Input: part model. Units: mm. Frame: model coordinates. Round coordinates to 2 decimals unless told otherwise and drop trailing zeros. Write each loop counter-clockwise with the first axis right and the second up, starting at its lowest first coordinate (ties: lowest second). Pieces come first, ordered by that corner, then holes. Notation, with made-up numbers: (-29.5, 12) -> (27.5, 12) arc R20 ccw to (27.5, 30) -> close; hole circle Ø11 at (-29.5, 34). An arc over 180 degrees is marked (long way). Use CSV: the item, a comma, the result in double quotes.
```python
from build123d import *

# Parameters (mm, degrees)
F0_W        = 21
F0_H        = 147
F1_DEPTH    = 4
F3_DEPTH    = 4.001
F4_T1_DEPTH = 171.4948974279


# Not quite as in the source:
# - a fillet or chamfer that OpenCascade refuses, or shapes differently, is made with other operations: its cross-section is extruded or revolved along the edge and cut away or added


with BuildPart() as f1:
    # F0 (on Top) → F1 (new body)
    with BuildSketch(Plane.XY):
        Rectangle(F0_W, F0_H)
    extrude(amount=F1_DEPTH)

    # F2 (on face) → F3 (cut, through all)
    with BuildSketch(Plane.XY.offset(4)):
        Polygon((10.5, 73.5), (-10.5, 73.5), (10.5, 52.5), align=None)
        Polygon((10.5, -52.5), (-10.5, -73.5), (10.5, -73.5), align=None)
    extrude(amount=-F3_DEPTH, mode=Mode.SUBTRACT)

    # F4: fillet of radius 5 on 1 edges, made by hand

    # F4_s2 → F4_t1 (cut)
    with BuildSketch(Plane.XZ.offset(-85.7474487139)):
        with BuildLine():
            ThreePointArc((-5.6010205144, 4), (-8.7632981746, 2.8729833462), (-10.5, 0))
            Line((-10.5, 0), (-10.5, 4))
            Line((-10.5, 4), (-5.6010205144, 4))
        make_face()
    extrude(amount=F4_T1_DEPTH, mode=Mode.SUBTRACT)


solid = f1.part
```
Item 1: Line query: line 1 (X direction, y = -54.5, z = 2.55); line 2 (Y direction, x = 4.5, z = 3.45); line 3 (Y direction, x = -3.5, z = 2.15). Output: solid intervals per line, ascending.
Worked answers:
line 1,"x = -9.12 to 8.5"
line 2,"y = -58.5 to 58.5"
line 3,"y = -66.5 to 66.5"
Item 2: First-contact query: pin 1 Ø1.5 at (x, z) = (7.5, 2.5) entering from -Y; pin 2 Ø5 at (x, y) = (1.5, 7) entering from -Z; pin 3 Ø1 at (y, z) = (-40, 3) entering from -X. Flat tips, straight axial feed; report the tip coordinate or a pass-through.
Worked answers:
pin 1,"stops at y = -56.25"
pin 2,"stops at z = 0"
pin 3,"stops at x = -9.17"
Item 3: Section query B-B on y = -13. Return the cut outline in (x, z).
Worked answers:
outline,"(-10.5, 0) -> (10.5, 0) -> (10.5, 4) -> (-5.6, 4) arc R5 ccw to start"
Item 4: Section query A-A on x = 2. Return the cut outline in (y, z), plus the area to 3 significant figures.
Worked answers:
outline,"(-61, 0) -> (61, 0) -> (61, 4) -> (-61, 4) -> close"
area,"488 mm²"
